Input: part model. Units: mm. Frame: model coordinates. A direction names the side the tool comes from. Give positions to 0.01 mm unless a question says otherwise; leave off trailing zeros. Order: outer loops, then holes, each group sorted by start corner. A loop starts at its lowest first (then second) coordinate and runs counter-clockwise, first axis right, second up. Notation, with made-up numbers: (83.25, 30) - (103.25, 30) arc R18 ccw to (103.25, 53) - close; hole circle Ø4 at (-36.75, 15.5). An arc over 180 degrees is marked (long way). Answer in a Markdown table with one row per item. Add a question column.
Autodesk Inventor part; units mm, degrees
ref_plane "YZ Plane" through (0, 0, 0) normal (1, 0, 0) x (0, 1, 0)
ref_plane "XZ Plane" through (0, 0, 0) normal (0, 1, 0) x (-1, 0, 0)
ref_plane "XY Plane" through (0, 0, 0) normal (0, 0, 1) x (1, 0, 0)
sketch "Sketch1" plane through (0, 0, 0) normal (0, 1, 0) x (-1, 0, 0)
  line L0 (0, 0) -> (53.4, 0)
  line L1 (5, -68.6) -> (2.3639, -65.9639)
  line L2 (5, -68.6) -> (8.728, -68.6) construction
  line L3 (2.3639, -65.9639) -> (0.3639, -65.9639)
  line L4 (0.3639, -65.9639) -> (0, -65.6)
  line L5 (52.7794, -66.2206) -> (53.4, -65.6)
  line L6 (52.7794, -66.2206) -> (40.7794, -66.2206)
  line L7 (40.7794, -66.2206) -> (37.9652, -68.6)
  line L8 (37.9652, -68.6) -> (5, -68.6)
  line L9 (53.4, -65.6) -> (53.4, 0)
  line L10 (0, 0) -> (0, -65.6)
  circle A0 centre (36.6794, -65.9103) radius 1.7
  circle A1 centre (6.3639, -65.6) radius 1.7
  dimension "d2" = 135
  dimension "d3" = 135
  dimension "d10" = 12
  dimension "d12" = 135
  dimension "d13" = 3.4
  dimension "d14" = 3.4
  dimension "d15" = 4.1
  dimension "d16" = 4
extrude "Extrusion1" add sketch "Sketch1" along normal blind 1.5
sketch "Sketch2" plane through (0, 1.5, 0) normal (0, 1, 0) x (1, 0, 0)
  circle A0 centre (-50.9, 14.75) radius 1.7
  line L0 (-53.4, 0) -> (0, 0)
  line L1 (-53.4, 65.6) -> (-53.4, 0)
  circle A1 centre (-2.5, 13.4) radius 1.7
  line L2 (0, 0) -> (0, 65.6)
  dimension "d19" = 3.4
  dimension "d20" = 14.75
  dimension "d21" = 2.5
  dimension "d22" = 3.4
  dimension "d23" = 13.4
  dimension "d24" = 2.5
extrude "Extrusion2" cut sketch "Sketch2" against normal blind 1.5
sketch "Sketch3" plane through (0, 1.5, 0) normal (0, 1, 0) x (1, 0, 0)
  line L0 (-1, 64.9639) -> (-3.3, 64.9639)
  line L1 (-3.3, 64.9639) -> (-3.3, 49.4639)
  line L2 (-3.3, 49.4639) -> (-1, 49.4639)
  line L3 (-1, 49.4639) -> (-1, 64.9639)
  line L4 (-0.3639, 65.9639) -> (-2.3639, 65.9639)
  line L5 (0, 0) -> (0, 65.6)
  line L6 (-3.3, 47.4639) -> (-1, 47.4639)
  line L7 (-1, 47.4639) -> (-1, 26.9639)
  line L8 (-1, 26.9639) -> (-3.3, 26.9639)
  line L9 (-3.3, 26.9639) -> (-3.3, 47.4639)
  line L10 (-52.4, 44.7206) -> (-50.1, 44.7206)
  line L11 (-50.1, 44.7206) -> (-50.1, 65.2206)
  line L12 (-50.1, 65.2206) -> (-52.4, 65.2206)
  line L13 (-52.4, 65.2206) -> (-52.4, 44.7206)
  line L14 (-53.4, 65.6) -> (-53.4, 0)
  line L15 (-40.7794, 66.2206) -> (-52.7794, 66.2206)
  line L16 (-52.4, 43.7206) -> (-50.1, 43.7206)
  line L17 (-50.1, 43.7206) -> (-50.1, 17.6206)
  line L18 (-50.1, 17.6206) -> (-52.4, 17.6206)
  line L19 (-52.4, 17.6206) -> (-52.4, 43.7206)
  dimension "d27" = 1
  dimension "d28" = 15.5
  dimension "d29" = 2.3
  dimension "d30" = 1
  dimension "d31" = 2
  dimension "d32" = 2.3
  dimension "d33" = 20.5
  dimension "d34" = 1
  dimension "d35" = 1
  dimension "d36" = 2.3
  dimension "d37" = 20.5
  dimension "d38" = 26.1
  dimension "d39" = 1
extrude "Extrusion3" add sketch "Sketch3" along normal blind 8.3
sketch "Sketch4" plane through (0, 1.5, 0) normal (0, 1, 0) x (1, 0, 0)
  line L0 (-20.8, 27.85) -> (-10.8, 27.85)
  line L1 (-10.8, 27.85) -> (-10.8, 63.6)
  line L2 (-10.8, 63.6) -> (-20.8, 63.6)
  line L3 (-20.8, 63.6) -> (-20.8, 27.85)
  line L4 (-3.3, 47.4639) -> (-3.3, 26.9639)
  line L5 (-5, 68.6) -> (-37.9652, 68.6)
  point P0 (0, 0)
  dimension "d42" = 10
  dimension "d43" = 35.75
  dimension "d44" = 7.5
  dimension "d45" = 5
extrude "Extrusion4" add sketch "Sketch4" along normal blind 8
chamfer "Chamfer1" distance 1 angle 45 2 edges at (-20.8, 9.5, -45.725) (-10.8, 9.5, -45.725)
sketch "Sketch5" plane through (0, 1.5, 0) normal (0, 1, 0) x (1, 0, 0)
  line L0 (-4.6091, 14.4286) -> (-11.1091, 14.4286)
  line L1 (-11.1091, 14.4286) -> (-11.1091, 20.9286)
  line L2 (-11.1091, 20.9286) -> (-4.6091, 20.9286)
  line L3 (-4.6091, 20.9286) -> (-4.6091, 14.4286)
  line L4 (-4.6091, 21.1286) -> (-11.1091, 21.1286)
  line L5 (-11.1091, 21.1286) -> (-11.1091, 27.6286)
  line L6 (-11.1091, 27.6286) -> (-4.6091, 27.6286)
  line L7 (-4.6091, 27.6286) -> (-4.6091, 21.1286)
  point P0 (0, 0)
  dimension "d51" = 6.5
  dimension "d52" = 6.5
  dimension "d53" = 6.5
  dimension "d54" = 0.2
extrude "Extrusion5" add sketch "Sketch5" along normal blind 2
sketch "Sketch6" plane through (0, 3.5, 0) normal (0, 1, 0) x (1, 0, 0)
  circle A0 centre (-7.8591, 17.6786) radius 3
  line L0 (-4.6091, 20.9286) -> (-11.1091, 20.9286)
  line L1 (-4.6091, 14.4286) -> (-4.6091, 20.9286)
  point P0 (0, 0)
  dimension "d57" = 6
  dimension "d58" = 3.25
  dimension "d59" = 3.25
extrude "Extrusion6" add sketch "Sketch6" along normal blind 3.6
sketch "Sketch7" plane through (0, 3.5, 0) normal (0, 1, 0) x (1, 0, 0)
  circle A0 centre (-7.8591, 24.3786) radius 3
  line L0 (-11.1091, 21.1286) -> (-4.6091, 21.1286)
  line L1 (-11.1091, 27.6286) -> (-11.1091, 21.1286)
  point P0 (0, 0)
  dimension "d62" = 6
  dimension "d63" = 3.25
  dimension "d64" = 3.25
extrude "Extrusion7" add sketch "Sketch7" along normal blind 3.6
fillet "Fillet1" radius 0.2 2 edges at (-10.8591, 7.1, -17.6786) (-10.8591, 7.1, -24.3786)
sketch "Sketch8" plane through (0, 1.5, 0) normal (0, 1, 0) x (1, 0, 0)
  line L0 (-52.8, 3) -> (-46.55, 3)
  line L1 (-46.55, 3) -> (-46.55, 9.25)
  line L2 (-46.55, 9.25) -> (-52.8, 9.25)
  line L3 (-52.8, 9.25) -> (-52.8, 3)
  line L4 (-53.4, 65.6) -> (-53.4, 0)
  line L5 (-53.4, 0) -> (0, 0)
  dimension "d68" = 6.25
  dimension "d69" = 6.25
  dimension "d70" = 0.6
  dimension "d71" = 3
extrude "Extrusion8" add sketch "Sketch8" along normal blind 1.5
sketch "Sketch9" plane through (0, 3, 0) normal (0, 1, 0) x (1, 0, 0)
  circle A0 centre (-49.8, 6) radius 1.5
  line L0 (-46.55, 9.25) -> (-52.8, 9.25)
  line L1 (-46.55, 3) -> (-46.55, 9.25)
  point P0 (0, 0)
  dimension "d74" = 3
  dimension "d75" = 3.25
  dimension "d76" = 3.25
extrude "Extrusion9" add sketch "Sketch9" along normal blind 1
sketch "Sketch10" plane through (0, 1.5, 0) normal (0, 1, 0) x (1, 0, 0)
  line L0 (-12.75, 0) -> (-3.75, 0)
  line L1 (-3.75, 0) -> (-3.75, 10)
  line L2 (-3.75, 10) -> (-12.75, 10)
  line L3 (-12.75, 10) -> (-12.75, 0)
  line L4 (0, 0) -> (0, 65.6)
  dimension "d79" = 9
  dimension "d80" = 10
  dimension "d81" = 3.75
extrude "Extrusion10" add sketch "Sketch10" along normal blind 10
sketch "Sketch11" plane through (-53.4, 0, 0) normal (0, 0, 1) x (1, 0, 0)
  line L0 (42.6, 1.5) -> (32.6, 1.5)
  line L1 (40.5024, 1.5) -> (49.871, 1.5)
  line L2 (49.871, 1.5) -> (49.871, 11.6818)
  line L3 (49.871, 11.6818) -> (40.5024, 11.6818)
  line L4 (40.5024, 11.6818) -> (40.5024, 1.5)
  point P0 (53.4, 0)
extrude "Extrusion11" add sketch "Sketch11" along normal blind 3.2
fillet "Fillet2" radius 4.5 2 edges at (-3.75, 11.5, -5) (-12.75, 11.5, -5)
sketch "Sketch12" plane through (-53.4, 0, 3.2) normal (0, 0, 1) x (1, 0, 0)
  circle A0 centre (45.1865, 6.591) radius 3.125
  line L0 (40.5024, 1.5) -> (49.871, 1.5)
  line L1 (49.871, 1.5) -> (49.871, 11.6818)
  point P0 (53.4, 0)
  dimension "d87" = 6.25
  dimension "d88" = 5.091
  dimension "d89" = 4.6845
extrude "Extrusion12" cut sketch "Sketch12" against normal blind 12
sketch "Sketch13" plane through (0, 1.5, 0) normal (0, 1, 0) x (1, 0, 0)
  line L0 (-44.5774, 0) -> (-32.5774, 0)
  line L1 (-32.5774, 0) -> (-32.5774, 8.75)
  line L2 (-32.5774, 8.75) -> (-44.5774, 8.75)
  line L3 (-44.5774, 8.75) -> (-44.5774, 0)
  point P0 (0, 0)
  dimension "d92" = 12
  dimension "d93" = 8.75
extrude "Extrusion13" add sketch "Sketch13" along normal blind 10.65
sketch "Sketch14" plane through (-53.4, 0, 0) normal (0, 0, 1) x (1, 0, 0)
  line L0 (8.8226, 1.5) -> (8.8226, 12.15)
  line L1 (48.4, 1.5) -> (15.4348, 1.5)
  line L2 (8.8226, 12.15) -> (20.8226, 12.15)
  line L3 (20.8226, 12.15) -> (20.8226, 1.5)
  line L4 (20.8226, 1.5) -> (8.8226, 1.5)
  line L5 (8.8226, 1.5) -> (8.8226, 12.15)
  point P0 (53.4, 0)
extrude "Extrusion14" add sketch "Sketch14" along normal blind 7
sketch "Sketch15" plane through (-53.4, 0, 7) normal (0, 0, 1) x (1, 0, 0)
  line L0 (19.3226, 3) -> (19.3226, 9.2358)
  line L1 (19.3226, 9.2358) -> (17.9084, 10.65)
  line L2 (17.9084, 10.65) -> (11.7368, 10.65)
  line L3 (11.7368, 10.65) -> (10.3226, 9.2358)
  line L4 (10.3226, 9.2358) -> (10.3226, 3)
  line L5 (10.3226, 3) -> (19.3226, 3)
  line L6 (20.8226, 1.5) -> (20.8226, 12.15)
  line L7 (8.8226, 12.15) -> (8.8226, 1.5)
  line L8 (20.8226, 12.15) -> (8.8226, 12.15)
  line L9 (8.8226, 1.5) -> (20.8226, 1.5)
  point P0 (53.4, 0)
  dimension "d98" = 2
  dimension "d99" = 135
  dimension "d100" = 2
  dimension "d101" = 135
  dimension "d102" = 1.5
  dimension "d103" = 1.5
  dimension "d104" = 1.5
  dimension "d105" = 1.5
extrude "Extrusion15" cut sketch "Sketch15" against normal blind 12 contours L5 L4 L3 L2 L1 L0
properties part number "arduinoUno"
Q1. Contact query for flat-ended pins moving along their axis: P1, Ø0.6, axis at x = -8, y = 2.5, coming from the +Z side; P2, Ø6.5, axis at y = 5.5, z = -50.5, coming from the +X side; P3, Ø0.6, axis at x = -6.5, y = 2.5, coming from the -Z side. Output: stop coordinate, or through.
Q2. Section B-B, the plane z = -48.5. Return loops of the section in (x, y), then the cut area to 3 significant figures.
Q3. Line query: probe 1 along X at (y, z) = (6.75, 1); probe 2 along X at (y, z) = (5.75, -52); probe 3 along X at (y, z) = (1, -65.6). Output: solid intervals per line, ascending.
Q4. Pull-direction query (Z, two-part tool) for faces 6 (the flat face through (-2, 6, -47.464)), 7 (the flat face through (-38, 7, -8.75)), 8 (the flat face through (-39, 10.65, 1)), 9 (the flat face through (-2, 6, -49.464)); classes: +Z half, -Z half, draft (parallel to the pull), parting line (faces both ways), or undercut.
Q5. Access query for faces 1 (the flat face through (-38, 1.5, 3)), 2 (the cylindrical face through (-5.103, 10.217, -5.07)), 3 (the flat face through (-50.1, 6, -31)), 4 (the flat face through (-11.109, 2, -18)), 5 (the flat face through (-50, 2, -9.25)). Directions: +Z, -Z, +X, -X, +Y, -Y. A direction counts if a zero-diameter tool reaches every point of the face in a straight line with its end or side. Return the directions, or none.
Q6. Section D-D, the plane z = -37. Return loops of the section in (x, y).
Q7. Section A-A, the plane z = -2. State how many separate pieces and enclosed holes the cut face has, then the cut area to 3 significant figures.
Computed:
| question | item | result |
|---|---|---|
| 1 | P1 | stops at z = 3.2 |
| 1 | P2 | stops at x = -1 |
| 1 | P3 | stops at z = -27.63 |
| 2 | outline | (-53.4, 0) - (0, 0) - (0, 1.5) - (-10.8, 1.5) - (-10.8, 8.5) - (-11.8, 9.5) - (-19.8, 9.5) - (-20.8, 8.5) - (-20.8, 1.5) - (-50.1, 1.5) - (-50.1, 9.8) - (-52.4, 9.8) - (-52.4, 1.5) - (-53.4, 1.5) - close |
| 2 | area | 178 mm^2 |
| 3 | probe 1 | x = -44.58 to -43.08, -34.08 to -32.58, -12.9 to -11.33, -5.09 to -3.53 |
| 3 | probe 2 | x = -52.4 to -50.1, -20.8 to -10.8, -3.3 to -1 |
| 3 | probe 3 | x = -53.4 to -38.35, -35.01 to -8.06, -4.66 to 0 |
| 4 | face 6 | undercut |
| 4 | face 7 | -Z half |
| 4 | face 8 | draft |
| 4 | face 9 | undercut |
| 5 | face 1 | +Z, +X, -X, -Y |
| 5 | face 2 | -Z, +X, +Y |
| 5 | face 3 | -Z, +Y |
| 5 | face 4 | +Y |
| 5 | face 5 | -X, +Y |
| 6 | outline | (-53.4, 0) - (0, 0) - (0, 1.5) - (-1, 1.5) - (-1, 9.8) - (-3.3, 9.8) - (-3.3, 1.5) - (-10.8, 1.5) - (-10.8, 8.5) - (-11.8, 9.5) - (-19.8, 9.5) - (-20.8, 8.5) - (-20.8, 1.5) - (-50.1, 1.5) - (-50.1, 9.8) - (-52.4, 9.8) - (-52.4, 1.5) - (-53.4, 1.5) - close |
| 7 | separate pieces | 1 |
| 7 | enclosed holes | 2 |
| 7 | area | 192 mm^2 |
